```python
from build123d import *

# Parameters (mm, degrees)
BOSS_EXTRUDE1_DEPTH = 5.842
FILLET1_R           = 12.7
FILLET2_R           = 1.5875


with BuildPart() as part:
    # Sketch1 → Boss-Extrude1 (new body)
    with BuildSketch(Plane(origin=(0, 0, 0), x_dir=(1, 0, 0), z_dir=(0, 1, 0))):
        Polygon((34.925, 0.357309717), (34.925, 4.964553254), (2.921, 12.7), (2.921, 6.35), (-2.921, 6.35), (-2.921, -6.35), (2.921, -6.35), (2.921, -9.525), align=None)
    extrude(amount=BOSS_EXTRUDE1_DEPTH)

    # Fillet1
    # the kernel refuses this fillet: 12.7 mm, written as the material it takes off along each edge
    with BuildSketch(Plane(origin=(34.925, -21.492812716, -4.964553254), x_dir=(0, 0, 1), z_dir=(0, 1, 0))) as fillet1_piece_1:
        with BuildLine():
            CenterArc((10.324747541, -11.340200526), FILLET1_R, 116.756334597, 49.655734511)
            Line((-2.019785945, -8.356495946), (-2.266676614, -8.296821854))
            Line((-2.266676614, -8.296821854), (-0.24689067, 0.059674092))
            Line((-0.24689067, 0.059674092), (0, 0.254))
            ThreePointArc((0, 0.254), (2.303621769, 0.254), (4.492893457, 0.226804011))
            Line((4.492893457, 0.226804011), (4.607243537, 0))
        make_face()
    extrude(amount=48.827625432, mode=Mode.SUBTRACT)

    # Fillet2
    fillet2_edges = [part.edges().sort_by_distance(p)[0] for p in [
        (34.925, 2.921, -0.357309717),
    ]]
    fillet(fillet2_edges, radius=FILLET2_R)


solid = part.part
```
Geometry: final body of the model. Coordinates: model frame, mm. A direction names the side the tool comes from. Coordinates: 2 decimals unless noted, no trailing zeros. Loops run counter-clockwise (first coordinate to the right, second up) from the corner with the lowest first, then second, coordinate; pieces in that order, holes last. Notation, with made-up numbers: M -30,86.25 L 29,86.25 A18 ccw 29,120.25 Z; hole C 30.25,-31.75 d3. An arc over 180 degrees is marked long. Put each result on its own line as item: value.
(1) First-contact query: pin 1 (3.5 mm diameter, centred on y = 3, z = 8.5, fed in from -X); pin 2 (3 mm diameter, centred on x = -0.5, y = 3, fed in from +Z); pin 3 (3 mm diameter, centred on x = 0.5, y = 2, fed in from -Z). Flat tips, straight axial feed; report the tip coordinate or a pass-through.
Answer sheet:
pin 1: stops at x = 2.92
pin 2: stops at z = 6.35
pin 3: stops at z = -6.35
(2) Material intervals for probe 1 along Z at (x, y) = (20.5, 3.65); probe 2 along Z at (x, y) = (9, 3); probe 3 along X at (y, z) = (4.2, -4), sorted ascending.
Answer sheet:
probe 1: z = -8.45 to 4.1
probe 2: z = -11.23 to 7.65
probe 3: x = -2.92 to 32.17
(3) Cut plane C-C on x = 19. Return the cut outline in (y, z), then the cut area to 3 significant figures.
Answer sheet:
outline: M 0,-8.81 L 5.84,-8.81 L 5.84,4.56 L 0,4.56 Z
area: 78.1 mm^2
(4) Cut plane B-B on z = -3.5. Return the cut outline in (x, y), then the cut area to 3 significant figures.
Answer sheet:
outline: M -2.92,0 L 32.68,0 L 32.68,5.84 L -2.92,5.84 Z
area: 208 mm^2
(5) Access query for faces 1 (the face through (0, 3, 6.35)), 2 (the face through (2.921, 3, -10)), 3 (the face through (30.64, 2.88, -5.2)). Directions: +Z, -Z, +X, -X, +Y, -Y. A direction counts if a zero-diameter tool reaches every point of the face in a straight line with its end or side. Return the directions, or none.
Answer sheet:
face 1: +Z, -X, +Y, -Y
face 2: -Z, -X, +Y, -Y
face 3: -Z, +X, +Y, -Y
